```python
from build123d import *

# Parameters (mm, degrees)
CROQUIS1_R              = 4
SALIENTE_EXTRUIR1_DEPTH = 260


with BuildPart() as part:
    # Croquis1 → Saliente-Extruir1 (new body)
    with BuildSketch(Plane(origin=(0, 0, 0), x_dir=(1, 0, 0), z_dir=(0, 1, 0))):
        with BuildLine():
            Line((-7, 15), (-15, 15))
            Line((-15, 15), (-15, 5.027604917))
            Line((-15, 5.027604917), (-12.623437069, 5.027604917))
            Line((-12.623437069, 5.027604917), (-12.623437069, 7.752682341))
            Line((-12.623437069, 7.752682341), (-11.320548438, 7.752682341))
            Line((-11.320548438, 7.752682341), (-7, 3.432133903))
            Line((-7, 3.432133903), (-7, -2.861090311))
            Line((-7, -2.861090311), (-12.793007796, -7))
            Line((-12.793007796, -7), (-13.527286117, -7))
            Line((-13.527286117, -7), (-13.527286117, -1.25796789))
            Line((-13.527286117, -1.25796789), (-15, -1.25796789))
            Line((-15, -1.25796789), (-15, -15))
            Line((-15, -15), (-3.139941254, -15))
            Line((-3.139941254, -15), (-3.139941254, -12.505835019))
            Line((-3.139941254, -12.505835019), (-6.77895709, -12.505835019))
            Line((-6.77895709, -12.505835019), (-6.77895709, -10.079824462))
            Line((-6.77895709, -10.079824462), (-2.512909638, -7.031876702))
            Line((-2.512909638, -7.031876702), (3.25590476, -7.031876702))
            Line((3.25590476, -7.031876702), (6.894920596, -10.079824462))
            Line((6.894920596, -10.079824462), (6.894920596, -12.505835019))
            Line((6.894920596, -12.505835019), (3.25590476, -12.505835019))
            Line((3.25590476, -12.505835019), (3.25590476, -15))
            Line((3.25590476, -15), (15, -15))
            Line((15, -15), (15, -7))
            ThreePointArc((15, -7), (8.556349186, 8.556349186), (-7, 15))
        make_face()
        Circle(CROQUIS1_R, mode=Mode.SUBTRACT)
    extrude(amount=SALIENTE_EXTRUIR1_DEPTH)


solid = part.part
```
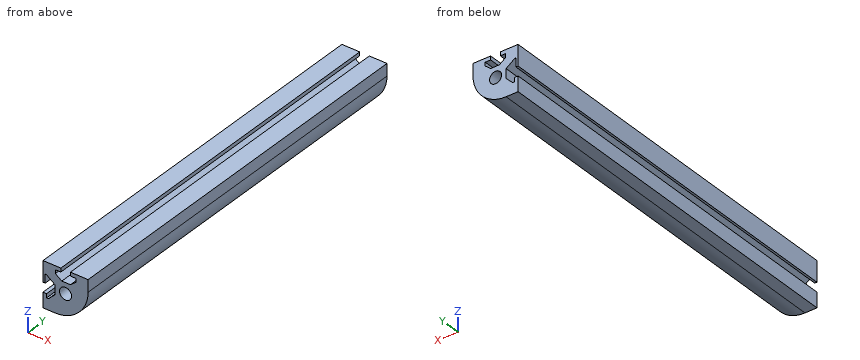
Source: CAD feature listing. Evaluate the final solid. Frame: model axes, mm. Coordinates: 2 decimals unless noted, no trailing zeros. Loops run counter-clockwise (first coordinate to the right, second up) from the corner with the lowest first, then second, coordinate; pieces in that order, holes last. Notation, with made-up numbers: (50.5, 14.5) -> (87.5, 14.5) arc R21 cw to (87.5, 46.5) -> close; hole circle Ø5 at (87, -32.5). An arc over 180 degrees is marked (long way). One line per item, written item: value. Start each with the question number.
Q1. Contact query for flat-ended pins moving along their axis: P1, Ø10, axis at y = 138.5, z = -4, coming from the +X side; P2, Ø3, axis at y = 85.5, z = -7, coming from the +X side; P3, Ø1.7, axis at x = 0.5, y = 126.5, coming from the +Z side. Output: stop coordinate, or through.
Q2. Line query: line 1 along X through (y, z) = (188, 13); line 2 along Z through (x, y) = (-3.5, 156); line 3 along Z through (x, y) = (0, 83). Output: solid intervals per line, ascending.
Q3. Section query B-B, the plane x = 0. Return the cut outline in (y, z).
Q4. Section query C-C, the plane x = 11.75. Return the cut outline in (y, z), and give its area (3 significant figures).
Q5. Section query A-A, the plane y = 69.5. Return the cut outline in (x, z).
Results:
1. P1: x = 14.17
1. P2: x = 11.1
1. P3: z = 7.03
2. line 1: -15 to -3.14, 3.26 to 15
2. line 2: -14.72 to -1.94, 1.94 to 7.74, 12.51 to 15
2. line 3: -13.86 to -4, 4 to 7.03
3. outline: (0, -13.86) -> (260, -13.86) -> (260, -4) -> (0, -4) -> close; (0, 4) -> (260, 4) -> (260, 7.03) -> (0, 7.03) -> close
4. outline: (0, -4.51) -> (260, -4.51) -> (260, 15) -> (0, 15) -> close
4. area: 5,070 mm^2
5. outline: (-15, -15) -> (-7, -15) arc R22 ccw to (15, 7) -> (15, 15) -> (3.26, 15) -> (3.26, 12.51) -> (6.89, 12.51) -> (6.89, 10.08) -> (3.26, 7.03) -> (-2.51, 7.03) -> (-6.78, 10.08) -> (-6.78, 12.51) -> (-3.14, 12.51) -> (-3.14, 15) -> (-15, 15) -> (-15, 1.26) -> (-13.53, 1.26) -> (-13.53, 7) -> (-12.79, 7) -> (-7, 2.86) -> (-7, -3.43) -> (-11.32, -7.75) -> (-12.62, -7.75) -> (-12.62, -5.03) -> (-15, -5.03) -> close; hole circle Ø8 at (0, 0)
